from build123d import *

# Parameters (mm, degrees)
CYLINDER081_R           = 1.6
CYLINDER081_DEPTH       = 40
CYLINDER081_PITCH_ANGLE = 90
CYLINDER077_R           = 1.6
CYLINDER077_DEPTH       = 40
CYLINDER077_PITCH_ANGLE = 90
CYLINDER076_R           = 1.6
CYLINDER076_DEPTH       = 40
CYLINDER076_PITCH_ANGLE = 90
CYLINDER080_R           = 1.6
CYLINDER080_DEPTH       = 40
CYLINDER080_PITCH_ANGLE = 90
CYLINDER079_R           = 1.6
CYLINDER079_DEPTH       = 40
CYLINDER079_PITCH_ANGLE = 90
CYLINDER078_R           = 1.6
CYLINDER078_DEPTH       = 40
CYLINDER078_PITCH_ANGLE = 90
BOX028_W                = 10
BOX028_H                = 22
BOX028_DEPTH            = 8
CYLINDER019_R           = 1.6
CYLINDER019_DEPTH       = 40
CYLINDER019_PITCH_ANGLE = 90
CYLINDER018_R           = 1.6
CYLINDER018_DEPTH       = 40
CYLINDER018_PITCH_ANGLE = 90
CYLINDER017_R           = 1.6
CYLINDER017_DEPTH       = 40
CYLINDER016_R           = 1.6
CYLINDER016_DEPTH       = 70
CYLINDER016_ROLL_ANGLE  = 90
CYLINDER015_R           = 1.6
CYLINDER015_DEPTH       = 40
BOX016_W                = 10
BOX016_H                = 8
BOX016_DEPTH            = 86
BOX014_W                = 5
BOX014_H                = 45
BOX014_DEPTH            = 154


with BuildPart() as cylinder359:
    # Cylinder081 → Cylinder081 (new body)
    with BuildSketch(Plane.XY):
        Circle(CYLINDER081_R)
    extrude(amount=CYLINDER081_DEPTH)


with BuildPart() as cylinder359_1:
    # Cylinder081 pitch: moved
    add(cylinder359.part.rotate(Axis((0, 0, 0), (0, 1, 0)), CYLINDER081_PITCH_ANGLE))


with BuildPart() as cylinder359_2:
    # Cylinder081 placement: moved
    add(cylinder359_1.part.moved(Location((-67, 7, 126))))


with BuildPart() as cylinder355:
    # Cylinder077 → Cylinder077 (new body)
    with BuildSketch(Plane.XY):
        Circle(CYLINDER077_R)
    extrude(amount=CYLINDER077_DEPTH)


with BuildPart() as cylinder355_1:
    # Cylinder077 pitch: moved
    add(cylinder355.part.rotate(Axis((0, 0, 0), (0, 1, 0)), CYLINDER077_PITCH_ANGLE))


with BuildPart() as cylinder355_2:
    # Cylinder077 placement: moved
    add(cylinder355_1.part.moved(Location((-67, -15, 30))))


with BuildPart() as rocker_screw_holes_d001:
    # Cylinder076 → Cylinder076 (new body)
    with BuildSketch(Plane.XY):
        Circle(CYLINDER076_R)
    extrude(amount=CYLINDER076_DEPTH)


with BuildPart() as rocker_screw_holes_d001_1:
    # Cylinder076 pitch: moved
    add(rocker_screw_holes_d001.part.rotate(Axis((0, 0, 0), (0, 1, 0)), CYLINDER076_PITCH_ANGLE))


with BuildPart() as rocker_screw_holes_d001_2:
    # Cylinder076 placement: moved
    add(rocker_screw_holes_d001_1.part.moved(Location((-87, -7, 30))))

    # Fusion051: union Cylinder355
    add(cylinder355_2.part)


with BuildPart() as rocker_screw_holes_d001_3:
    # Fusion051 placement: moved
    add(rocker_screw_holes_d001_2.part.moved(Location((0, 0, 96))))

    # Fusion054: union Cylinder359
    add(cylinder359_2.part)


with BuildPart() as cylinder358:
    # Cylinder080 → Cylinder080 (new body)
    with BuildSketch(Plane.XY):
        Circle(CYLINDER080_R)
    extrude(amount=CYLINDER080_DEPTH)


with BuildPart() as cylinder358_1:
    # Cylinder080 pitch: moved
    add(cylinder358.part.rotate(Axis((0, 0, 0), (0, 1, 0)), CYLINDER080_PITCH_ANGLE))


with BuildPart() as cylinder358_2:
    # Cylinder080 placement: moved
    add(cylinder358_1.part.moved(Location((-67, 7, 30))))


with BuildPart() as cylinder357:
    # Cylinder079 → Cylinder079 (new body)
    with BuildSketch(Plane.XY):
        Circle(CYLINDER079_R)
    extrude(amount=CYLINDER079_DEPTH)


with BuildPart() as cylinder357_1:
    # Cylinder079 pitch: moved
    add(cylinder357.part.rotate(Axis((0, 0, 0), (0, 1, 0)), CYLINDER079_PITCH_ANGLE))


with BuildPart() as cylinder357_2:
    # Cylinder079 placement: moved
    add(cylinder357_1.part.moved(Location((-67, -15, 30))))


with BuildPart() as rocker_screw_holes_c001:
    # Cylinder078 → Cylinder078 (new body)
    with BuildSketch(Plane.XY):
        Circle(CYLINDER078_R)
    extrude(amount=CYLINDER078_DEPTH)


with BuildPart() as rocker_screw_holes_c001_1:
    # Cylinder078 pitch: moved
    add(rocker_screw_holes_c001.part.rotate(Axis((0, 0, 0), (0, 1, 0)), CYLINDER078_PITCH_ANGLE))


with BuildPart() as rocker_screw_holes_c001_2:
    # Cylinder078 placement: moved
    add(rocker_screw_holes_c001_1.part.moved(Location((-87, -7, 30))))

    # Fusion052: union Cylinder357
    add(cylinder357_2.part)

    # Fusion053: union Cylinder358
    add(cylinder358_2.part)


with BuildPart() as cube016:
    # Box028 → Box028 (new body)
    with BuildSketch(Plane(origin=(-37, -18, 18), x_dir=(1, 0, 0), z_dir=(0, 0, 1))):
        with Locations((5, 11)):
            Rectangle(BOX028_W, BOX028_H)
    extrude(amount=BOX028_DEPTH)


with BuildPart() as cylinder100:
    # Cylinder019 → Cylinder019 (new body)
    with BuildSketch(Plane.XY):
        Circle(CYLINDER019_R)
    extrude(amount=CYLINDER019_DEPTH)


with BuildPart() as cylinder100_1:
    # Cylinder019 pitch: moved
    add(cylinder100.part.rotate(Axis((0, 0, 0), (0, 1, 0)), CYLINDER019_PITCH_ANGLE))


with BuildPart() as cylinder100_2:
    # Cylinder019 placement: moved
    add(cylinder100_1.part.moved(Location((-40, 12, 9.5))))


with BuildPart() as fusion011:
    # Cylinder018 → Cylinder018 (new body)
    with BuildSketch(Plane.XY):
        Circle(CYLINDER018_R)
    extrude(amount=CYLINDER018_DEPTH)


with BuildPart() as fusion011_1:
    # Cylinder018 pitch: moved
    add(fusion011.part.rotate(Axis((0, 0, 0), (0, 1, 0)), CYLINDER018_PITCH_ANGLE))


with BuildPart() as fusion011_2:
    # Cylinder018 placement: moved
    add(fusion011_1.part.moved(Location((-40, -7, 2.5))))

    # Fusion011: union Cylinder100
    add(cylinder100_2.part)


with BuildPart() as fusion012:
    # Cylinder017 → Cylinder017 (new body)
    with BuildSketch(Plane(origin=(-27.5, 7, -15), x_dir=(1, 0, 0), z_dir=(0, 0, 1))):
        Circle(CYLINDER017_R)
    extrude(amount=CYLINDER017_DEPTH)

    # Fusion012: union Fusion011
    add(fusion011_2.part)


with BuildPart() as fusion013:
    # Cylinder016 → Cylinder016 (new body)
    with BuildSketch(Plane.XY):
        Circle(CYLINDER016_R)
    extrude(amount=CYLINDER016_DEPTH)


with BuildPart() as fusion013_1:
    # Cylinder016 roll: moved
    add(fusion013.part.rotate(Axis((0, 0, 0), (1, 0, 0)), CYLINDER016_ROLL_ANGLE))


with BuildPart() as fusion013_2:
    # Cylinder016 placement: moved
    add(fusion013_1.part.moved(Location((-24, 39, 6))))

    # Fusion013: union Fusion012
    add(fusion012.part)


with BuildPart() as cylinder008:
    # Cylinder015 → Cylinder015 (new body)
    with BuildSketch(Plane(origin=(-20.5, -12, -15), x_dir=(1, 0, 0), z_dir=(0, 0, 1))):
        Circle(CYLINDER015_R)
    extrude(amount=CYLINDER015_DEPTH)


with BuildPart() as face_corner_holes010:
    # Fusion024 base: copy of Cylinder008
    add(cylinder008.part)

    # Fusion024: union Fusion013
    add(fusion013_2.part)


with BuildPart() as face_corner_holes010_1:
    # Fusion024 placement: moved
    add(face_corner_holes010.part.moved(Location((0, 0, 132))))


with BuildPart() as face_corner_holes:
    # Fusion014 base: copy of Cylinder008
    add(cylinder008.part)

    # Fusion014: union Fusion013
    add(fusion013_2.part)


with BuildPart() as string_hole:
    # Box016 → Box016 (new body)
    with BuildSketch(Plane(origin=(-36, -15, 35), x_dir=(1, 0, 0), z_dir=(0, 0, 1))):
        with Locations((5, 4)):
            Rectangle(BOX016_W, BOX016_H)
    extrude(amount=BOX016_DEPTH)


with BuildPart() as bottom_a:
    # Box014 → Box014 (new body)
    with BuildSketch(Plane(origin=(-35, -23, -5), x_dir=(1, 0, 0), z_dir=(0, 0, 1))):
        with Locations((2.5, 22.5)):
            Rectangle(BOX014_W, BOX014_H)
    extrude(amount=BOX014_DEPTH)

    # Cut007: cut string-hole
    add(string_hole.part, mode=Mode.SUBTRACT)

    # Cut012: cut face-corner-holes
    add(face_corner_holes.part, mode=Mode.SUBTRACT)

    # Cut021: cut face-corner-holes010
    add(face_corner_holes010_1.part, mode=Mode.SUBTRACT)

    # Cut034: cut Cube016
    add(cube016.part, mode=Mode.SUBTRACT)

    # Cut043: cut rocker-screw-holes-c001
    add(rocker_screw_holes_c001_2.part, mode=Mode.SUBTRACT)

    # Cut044: cut rocker-screw-holes-d001
    add(rocker_screw_holes_d001_3.part, mode=Mode.SUBTRACT)


solid = bottom_a.part
Could you check a few things on this model? Use its own coordinates, in mm. A direction names the side the tool comes from. Coordinates: 2 decimals unless noted, no trailing zeros. Order: outer loops, then holes, each group sorted by start corner. A loop starts at its lowest first (then second) coordinate and runs counter-clockwise, first axis right, second up. Notation, with made-up numbers: (-7.75, 54.5) -> (49.25, 54.5) arc R20 cw to (49.25, 75.5) -> close; hole circle Ø2 at (67, -27). An arc over 180 degrees is marked (long way). One line per item, written item: value. Start each with the question number.
1) If I drill on L1, parallel to Z at x = -30.65, y = -12; L2, parallel to Y at x = -33.05, z = 30; L3, parallel to Z at x = -33, y = 12, over which ranges is the centre line in solid material (lowest first)? Write a range as [from, to].
2) We'd pull the mould along Y, two halves only. Please class faces 1 (the flat face through (-33, -23, 71)), 2 (the flat face through (-33, 0, -5)), 3 (the cylindrical face through (-32.53, 11.39, 140.02)), 4 (the cylindrical face through (-32.53, -8.56, 2.85)): +Y half, -Y half, draft (parallel to the pull), parting line (faces both ways), or undercut.
3) Which directions (+Z, -Z, +X, -X, +Y, -Y) give clear straight access to the entire face, cutting with the end or side of a thin tool? Please do faces 5 (the flat face through (-33, -11, 121)), 6 (the flat face through (-33, 22, 71)).
4) Imagine slicing it at B-B on z = 99.5. List the corners of the cut face in (x, y) for me, plus the area to 3 significant figures.
5) Imagine slicing it at C-C on z = 30. List the corners of the cut face in (x, y) for me.
6) Imagine slicing it at A-A on y = 12. List the corners of the cut face in (x, z) for me, plus the area to 3 significant figures.
7) I'm going to push a flat-ended pin straight in: pin 1 (1.9 mm diameter, centred on y = -7, z = 2.5, fed in from -X). Where does the tip first touch, or does it pass through?
8) Imagine slicing it at D-D on x = -34.1. Count the separate pieces of the cut face and the enclosed holes in it, plus the area to 3 significant figures.
Answer list:
1. L1: z = [-5, 18], [26, 35], [121, 149]
1. L2: y = [-23, -16.6], [-13.4, 5.4], [8.6, 22]
1. L3: z = [-5, 7.9], [11.1, 139.9], [143.1, 149]
2. face 1: -Y half
2. face 2: draft
2. face 3: undercut
2. face 4: undercut
3. face 5: +X, -X
3. face 6: +Z, -Z, +X, -X, +Y
4. outline: (-35, -23) -> (-30, -23) -> (-30, -15) -> (-35, -15) -> close; (-35, -7) -> (-30, -7) -> (-30, 22) -> (-35, 22) -> close
4. area: 185 mm2
5. outline: (-35, -23) -> (-30, -23) -> (-30, -16.6) -> (-35, -16.6) -> close; (-35, -13.4) -> (-30, -13.4) -> (-30, 5.4) -> (-35, 5.4) -> close; (-35, 8.6) -> (-30, 8.6) -> (-30, 22) -> (-35, 22) -> close
6. outline: (-35, -5) -> (-30, -5) -> (-30, 7.9) -> (-35, 7.9) -> close; (-35, 11.1) -> (-30, 11.1) -> (-30, 139.9) -> (-35, 139.9) -> close; (-35, 143.1) -> (-30, 143.1) -> (-30, 149) -> (-35, 149) -> close
6. area: 738 mm2
7. pin 1: passes through
8. separate pieces: 1
8. enclosed holes: 10
8. area: 6,000 mm2
